Autodesk Inventor part; units mm, degrees
ref_plane "YZ Plane" through (0, 0, 0) normal (1, 0, 0) x (0, 1, 0)
ref_plane "XZ Plane" through (0, 0, 0) normal (0, 1, 0) x (-1, 0, 0)
ref_plane "XY Plane" through (0, 0, 0) normal (0, 0, 1) x (1, 0, 0)
sketch "Sketch1" plane through (0, 0, 0) normal (0, 0, 1) x (1, 0, 0)
  circle A0 centre (-14, 16.5) radius 1.5
  circle A1 centre (14, 16.5) radius 1.5
  line L0 (-12, 0) -> (-12, 14.5)
  line L1 (-12, 14.5) -> (12, 14.5)
  line L2 (12, 14.5) -> (12, 0)
  line L3 (12, 0) -> (17, 0)
  line L4 (17, 0) -> (17, 17.5)
  line L5 (15, 19.5) -> (17, 17.5)
  line L6 (-15, 19.5) -> (15, 19.5)
  line L7 (-17, 17.5) -> (-15, 19.5)
  line L8 (-17, 0) -> (-17, 17.5)
  line L9 (-17, 0) -> (-12, 0)
  line L10 (0, 14.5) -> (0, 0)
  circle A2 centre (-14, -16.5) radius 1.5
  circle A3 centre (14, -16.5) radius 1.5
  line L11 (-12, 0) -> (-12, -14.5)
  line L12 (-12, -14.5) -> (12, -14.5)
  line L13 (12, -14.5) -> (12, 0)
  line L14 (17, 0) -> (17, -17.5)
  line L15 (15, -19.5) -> (17, -17.5)
  line L16 (-15, -19.5) -> (15, -19.5)
  line L17 (-17, -17.5) -> (-15, -19.5)
  line L18 (-17, 0) -> (-17, -17.5)
  line L19 (0, -14.5) -> (0, 0)
  point P0 (0, 0)
  point P1 (0, 12)
  point P2 (0, -12)
extrude "Extrusion1" add sketch "Sketch1" along normal blind 3
chamfer "Chamfer1" distance 1 angle 45 8 edges at (-16, -18.5, 3) (-16, 18.5, 3) (16, 18.5, 3) (16, -18.5, 3) (0, -19.5, 3) (0, 19.5, 3) (-17, 8.75, 3) (17, 8.75, 3)
properties part number "manta ray handle cap"
Read the model definition and answer for the solid it produces. Units are mm, in the model's axes. Give positions to 0.01 mm unless a question says otherwise; leave off trailing zeros. Order: outer loops, then holes, each group sorted by start corner. A loop starts at its lowest first (then second) coordinate and runs counter-clockwise, first axis right, second up. Notation, with made-up numbers: (53, 36.5) -> (74, 36.5) arc R16 ccw to (74, 44.5) -> close; hole circle Ø8 at (59, 72.25). An arc over 180 degrees is marked (long way). Write item = value, one per line.
1. A cutting plane is placed at B-B, the plane y = 16.5. Write down the section's boundary in (x, z), and give its area (3 significant figures).
Numbers:
outline = (-17, 0) -> (-15.5, 0) -> (-15.5, 3) -> (-16, 3) -> (-17, 2) -> close; (-12.5, 0) -> (12.5, 0) -> (12.5, 3) -> (-12.5, 3) -> close; (15.5, 0) -> (17, 0) -> (17, 2) -> (16, 3) -> (15.5, 3) -> close
area = 83.0 mm²
2. A cutting plane is placed at A-A, the plane x = 14. Write down the section's boundary in (y, z), and give its area (3 significant figures).
Numbers:
outline = (-19.5, 0) -> (-18, 0) -> (-18, 3) -> (-18.5, 3) -> (-19.5, 2) -> close; (-15, 0) -> (15, 0) -> (15, 3) -> (-15, 3) -> close; (18, 0) -> (19.5, 0) -> (19.5, 2) -> (18.5, 3) -> (18, 3) -> close
area = 98.0 mm²
3. The mould has two halves that part along Y. Classify faces 1 (the face through (0, 19.5, 1)), 2 (the face through (-15.11, -17.51, 1.48)), 3 (the face through (-15.5, 16.43, 1.48)), 4 (the face through (15.64, -18.17, 2.49)): +Y half, -Y half, draft (parallel to the pull), parting line (faces both ways), or undercut.
Numbers:
face_1 = +Y half
face_2 = undercut
face_3 = undercut
face_4 = -Y half
4. A cutting plane is placed at C-C, the plane z = 1.5. Write down the section's boundary in (x, y), and give its area (3 significant figures).
Numbers:
outline = (-17, -17.5) -> (-15, -19.5) -> (15, -19.5) -> (17, -17.5) -> (17, 17.5) -> (15, 19.5) -> (-15, 19.5) -> (-17, 17.5) -> close; hole circle Ø3 at (-14, -16.5); hole circle Ø3 at (-14, 16.5); hole circle Ø3 at (14, -16.5); hole circle Ø3 at (14, 16.5)
area = 1,290 mm²
5. Given pin 1 (2.5 mm diameter, centred on x = 14, y = -16.5, fed in from +Z), flat-ended and moving along its own axis, determine where the tip first touches the part or whether it passes through.
Numbers:
pin_1 = through
6. Straight lines are drawn through the part: line 1 along Y through (x, z) = (-14, 0.7); line 2 along Y through (x, z) = (15, 1.9); line 3 along X through (y, z) = (-15.5, 0.45). For each, find the intervals that lie inside material, in ascending order.
Numbers:
line_1 = -19.5 to -18, -15 to 15, 18 to 19.5
line_2 = -19.5 to -17.62, -15.38 to 15.38, 17.62 to 19.5
line_3 = -17 to -15.12, -12.88 to 12.88, 15.12 to 17
